from build123d import *

# Parameters (mm, degrees)
SKETCH1_R                                         = 10.25
BOSS_EXTRUDE1_DEPTH                               = 0.8
CSK_FOR_M2_5_FLAT_HEAD_MACHINE_SCREW1_D           = 2.9
CSK_FOR_M2_5_FLAT_HEAD_MACHINE_SCREW1_DEPTH       = 15
CSK_FOR_M2_5_FLAT_HEAD_MACHINE_SCREW1_CSINK_D     = 5.5
CSK_FOR_M2_5_FLAT_HEAD_MACHINE_SCREW1_CSINK_ANGLE = 90
CSK_FOR_M2_5_FLAT_HEAD_MACHINE_SCREW1_TIP         = 0.871247898
SKETCH2_R                                         = 1.75
CUT_EXTRUDE1_DEPTH                                = 0.5
SKETCH5_R                                         = 0.775
CUT_EXTRUDE2_DEPTH                                = 0.5
BOSS_EXTRUDE2_START                               = 1
SKETCH6_R                                         = 10.25
SKETCH6_R_2                                       = 1.75
SKETCH6_R_3                                       = 2.75
BOSS_EXTRUDE2_DEPTH                               = 1
CUT_EXTRUDE3_DEPTH                                = 1
CUT_EXTRUDE4_DEPTH                                = 1


with BuildPart() as part:
    # Sketch1 → Boss-Extrude1 (new body)
    with BuildSketch(Plane(origin=(0, 0, 0), x_dir=(1, 0, 0), z_dir=(0, 1, 0))):
        with Locations(Location((0, 0, 0), (0, 0, 270))):
            Circle(SKETCH1_R)
    extrude(amount=BOSS_EXTRUDE1_DEPTH)

    # CSK for M2.5 Flat Head Machine Screw1
    with Locations(Plane(origin=(0, 0.8, 0), x_dir=(1, 0, 0), z_dir=(0, 1, 0))):
        with Locations((0, 0)):
            CounterSinkHole(CSK_FOR_M2_5_FLAT_HEAD_MACHINE_SCREW1_D / 2, CSK_FOR_M2_5_FLAT_HEAD_MACHINE_SCREW1_CSINK_D / 2, depth=CSK_FOR_M2_5_FLAT_HEAD_MACHINE_SCREW1_DEPTH, counter_sink_angle=CSK_FOR_M2_5_FLAT_HEAD_MACHINE_SCREW1_CSINK_ANGLE)
            with Locations((0, 0, -(CSK_FOR_M2_5_FLAT_HEAD_MACHINE_SCREW1_DEPTH + CSK_FOR_M2_5_FLAT_HEAD_MACHINE_SCREW1_TIP / 2))):  # 118° drill point
                Cone(0, CSK_FOR_M2_5_FLAT_HEAD_MACHINE_SCREW1_D / 2, CSK_FOR_M2_5_FLAT_HEAD_MACHINE_SCREW1_TIP, mode=Mode.SUBTRACT)

    # Sketch2 → Cut-Extrude1 (cut)
    with BuildSketch(Plane(origin=(0, 0.8, 0), x_dir=(1, 0, 0), z_dir=(0, 1, 0))):
        with Locations(Location((-4.610336213, -4.610336213, 0), (0, 0, 270))):
            Circle(SKETCH2_R)
        with Locations(Location((4.610336213, 4.610336213, 0), (0, 0, 270))):
            Circle(SKETCH2_R)
        with Locations(Location((4.610336213, -4.610336213, 0), (0, 0, 270))):
            Circle(SKETCH2_R)
        with Locations(Location((-4.610336213, 4.610336213, 0), (0, 0, 270))):
            Circle(SKETCH2_R)
    extrude(amount=-CUT_EXTRUDE1_DEPTH, mode=Mode.SUBTRACT)

    # Sketch5 → Cut-Extrude2 (cut)
    with BuildSketch(Plane(origin=(0, 0.3, 0), x_dir=(1, 0, 0), z_dir=(0, 1, 0))):
        with Locations(Location((-4.610336213, -4.610336213, 0), (0, 0, 270))):
            Circle(SKETCH5_R)
        with Locations(Location((4.610336213, 4.610336213, 0), (0, 0, 270))):
            Circle(SKETCH5_R)
        with Locations(Location((4.610336213, -4.610336213, 0), (0, 0, 270))):
            Circle(SKETCH5_R)
        with Locations(Location((-4.610336213, 4.610336213, 0), (0, 0, 270))):
            Circle(SKETCH5_R)
    extrude(amount=-CUT_EXTRUDE2_DEPTH, mode=Mode.SUBTRACT)

    # Sketch6 → Boss-Extrude2 (add)
    with BuildSketch(Plane(origin=(0, 0.8, 0), x_dir=(1, 0, 0), z_dir=(0, 1, 0)).offset(BOSS_EXTRUDE2_START)):
        with Locations(Location((0, 0, 0), (0, 0, 270))):
            Circle(SKETCH6_R)
        with Locations(Location((4.610336213, 4.610336213, 0), (0, 0, 270))):
            Circle(SKETCH6_R_2, mode=Mode.SUBTRACT)
        with Locations(Location((0, 0, 0), (0, 0, 270))):
            Circle(SKETCH6_R_3, mode=Mode.SUBTRACT)
        with Locations(Location((-4.610336213, -4.610336213, 0), (0, 0, 270))):
            Circle(SKETCH6_R_2, mode=Mode.SUBTRACT)
        with Locations(Location((4.610336213, -4.610336213, 0), (0, 0, 270))):
            Circle(SKETCH6_R_2, mode=Mode.SUBTRACT)
        with Locations(Location((-4.610336213, 4.610336213, 0), (0, 0, 270))):
            Circle(SKETCH6_R_2, mode=Mode.SUBTRACT)
    extrude(amount=-BOSS_EXTRUDE2_DEPTH)

    # Sketch12 → Cut-Extrude3 (cut)
    with BuildSketch(Plane.XZ):
        with BuildLine():
            Line((-3.21438925, 7.852976026), (-2.257680669, 5.543277195))
            ThreePointArc((-2.257680669, 5.543277195), (0.038419926, 6), (2.33452052, 5.543277195))
            Line((2.33452052, 5.543277195), (3.291229101, 7.852976026))
            ThreePointArc((3.291229101, 7.852976026), (0.038419926, 8.5), (-3.21438925, 7.852976026))
        make_face()
        with BuildLine():
            Line((-5.50485727, 2.296100594), (-7.814556101, 3.252809175))
            ThreePointArc((-7.814556101, 3.252809175), (-8.461580074, 0), (-7.814556101, -3.252809175))
            Line((-7.814556101, -3.252809175), (-5.50485727, -2.296100594))
            ThreePointArc((-5.50485727, -2.296100594), (-5.961580074, 0), (-5.50485727, 2.296100594))
        make_face()
        with BuildLine():
            Line((-2.257680669, -5.543277195), (-3.21438925, -7.852976026))
            ThreePointArc((-3.21438925, -7.852976026), (0.038419926, -8.5), (3.291229101, -7.852976026))
            Line((3.291229101, -7.852976026), (2.33452052, -5.543277195))
            ThreePointArc((2.33452052, -5.543277195), (0.038419926, -6), (-2.257680669, -5.543277195))
        make_face()
        with BuildLine():
            Line((7.891395952, 3.252809175), (5.581697121, 2.296100594))
            ThreePointArc((5.581697121, 2.296100594), (6.038419926, 0), (5.581697121, -2.296100594))
            Line((5.581697121, -2.296100594), (7.891395952, -3.252809175))
            ThreePointArc((7.891395952, -3.252809175), (8.538419926, 0), (7.891395952, 3.252809175))
        make_face()
    extrude(amount=-CUT_EXTRUDE3_DEPTH, mode=Mode.SUBTRACT)

    # Sketch13 → Cut-Extrude4 (cut)
    with BuildSketch(Plane(origin=(0, 0, 0), x_dir=(-1, 0, 0), z_dir=(0, -1, 0))):
        with BuildLine():
            Line((2.32440044, 4.984692829), (3.803564356, 8.156770083))
            ThreePointArc((3.803564356, 8.156770083), (0, 9), (-3.803564356, 8.156770083))
            Line((-3.803564356, 8.156770083), (-2.32440044, 4.984692829))
            ThreePointArc((-2.32440044, 4.984692829), (0, 5.5), (2.32440044, 4.984692829))
        make_face()
        with BuildLine():
            Line((4.984692829, 2.32440044), (8.156770083, 3.803564356))
            ThreePointArc((8.156770083, 3.803564356), (9, 0), (8.156770083, -3.803564356))
            Line((8.156770083, -3.803564356), (4.984692829, -2.32440044))
            ThreePointArc((4.984692829, -2.32440044), (5.5, 0), (4.984692829, 2.32440044))
        make_face()
        with BuildLine():
            Line((2.32440044, -4.984692829), (3.803564356, -8.156770083))
            ThreePointArc((3.803564356, -8.156770083), (0, -9), (-3.803564356, -8.156770083))
            Line((-3.803564356, -8.156770083), (-2.32440044, -4.984692829))
            ThreePointArc((-2.32440044, -4.984692829), (0, -5.5), (2.32440044, -4.984692829))
        make_face()
        with BuildLine():
            Line((-4.984692829, -2.32440044), (-8.156770083, -3.803564356))
            ThreePointArc((-8.156770083, -3.803564356), (-9, 0), (-8.156770083, 3.803564356))
            Line((-8.156770083, 3.803564356), (-4.984692829, 2.32440044))
            ThreePointArc((-4.984692829, 2.32440044), (-5.5, 0), (-4.984692829, -2.32440044))
        make_face()
    extrude(amount=-CUT_EXTRUDE4_DEPTH, mode=Mode.SUBTRACT)


solid = part.part
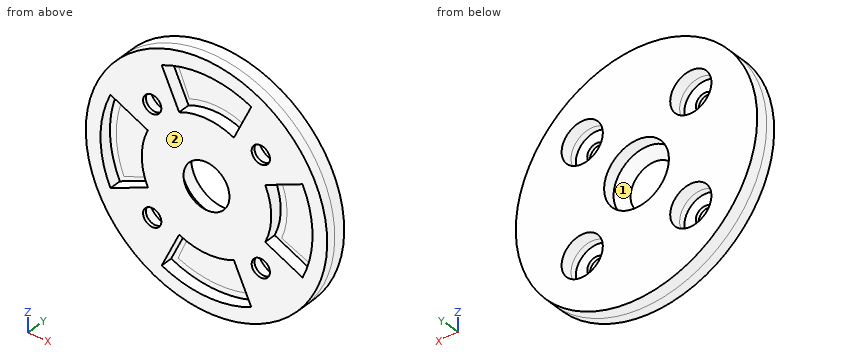
Verification items for the finished model (mm, model axes). Face numbers are marked on the shaded views. Give positions to 0.01 mm unless a question says otherwise; leave off trailing zeros. Write each loop counter-clockwise with the first axis right and the second up, starting at its lowest first coordinate (ties: lowest second). Pieces come first, ordered by that corner, then holes. Notation, with made-up numbers: M 21.25,82 L 51.25,82 A24 ccw 51.25,104 Z; hole C 18,-27 d8. An arc over 180 degrees is marked long. Write item = value, one per line.
(1) Sectioned sample at C-C (y = 1.35). Record the cut outline in (x, z).
Found:
outline = C 0,0 d20.5; hole C -4.61,-4.61 d3.5; hole C -4.61,4.61 d3.5; hole C 0,0 d5.5; hole C 4.61,-4.61 d3.5; hole C 4.61,4.61 d3.5
(2) Material ranges on line 1 (Z direction, x = 5, y = 1.05); line 2 (Z direction, x = -1.75, y = 0.35); line 3 (X direction, y = 0.85, z = 3.5), recorded low to high.
Found:
line_1 = -8.95 to -6.32, -2.9 to 2.9, 6.32 to 8.95
line_2 = -10.1 to -8.83, -5.21 to -1.49, 1.49 to 5.21, 8.83 to 10.1
line_3 = -9.63 to -8.29, -7.51 to -5.96, -3.26 to 3.26, 5.96 to 7.51, 8.29 to 9.63
(3) Sectioned sample at A-A (x = 0). Record the cut outline in (y, z), then the cut area to 3 significant figures.
Found:
outline = M 0,-10.25 L 1.8,-10.25 L 1.8,-2.75 L 0.8,-2.75 L 0,-1.95 L 0,-5.5 L 1,-5.5 L 1,-9 L 0,-9 Z; M 0,1.95 L 0.8,2.75 L 1.8,2.75 L 1.8,10.25 L 0,10.25 L 0,9 L 1,9 L 1,5.5 L 0,5.5 Z
area = 20.6 mm2
(4) Sectioned sample at D-D (x = -5.75). Record the cut outline in (y, z), then the cut area to 3 significant figures.
Found:
outline = M 0,-8.49 L 1.8,-8.49 L 1.8,-5.94 L 0.3,-5.94 L 0.3,-3.28 L 1.8,-3.28 L 1.8,3.28 L 0.3,3.28 L 0.3,5.94 L 1.8,5.94 L 1.8,8.49 L 0,8.49 L 0,2.68 L 1,2.68 L 1,-2.68 L 0,-2.68 Z
area = 17.2 mm2
(5) Go/stop test with flat-tipped pins: pin 1 Ø1 at (x, y) = (-7, 0.5) entering from +Z; pin 2 Ø1.4 at (x, z) = (4.61, 4.61) entering from +Y; pin 3 Ø3 at (x, z) = (-4.61, 4.61) entering from +Y; pin 4 Ø2.5 at (x, z) = (1.5, -7.5) entering from -Y. Record where each tip stops, or that it passes through.
Found:
pin_1 = 7.93
pin_2 = through
pin_3 = 0.3
pin_4 = 1
(6) Sectioned sample at B-B (z = 0). Record the cut outline in (x, y), then the cut area to 3 significant figures.
Found:
outline = M -10.25,0 L -9,0 L -9,1 L -5.5,1 L -5.5,0 L -1.95,0 L -2.75,0.8 L -2.75,1.8 L -10.25,1.8 Z; M 1.95,0 L 5.5,0 L 5.5,1 L 9,1 L 9,0 L 10.25,0 L 10.25,1.8 L 2.75,1.8 L 2.75,0.8 Z
area = 20.6 mm2
(7) Draft check along X on the marked faces 1 and 2. Enter one of: released by +X, released by -X, zero draft, split by the parting line, or undercut.
Found:
face_1 = undercut
face_2 = zero draft
